Check sheet for the modelled part. Datum: model origin and axes. Units: mm. A direction names the side the tool comes from. Round coordinates to 2 decimals unless told otherwise and drop trailing zeros. Order: outer loops, then holes, each group sorted by start corner. A loop starts at its lowest first (then second) coordinate and runs counter-clockwise, first axis right, second up.
Q1. Cross-section at A-A on y = 2.1. Record the cut outline in (x, z), then the cut area to 3 significant figures.
Q2. Set-up check for faces 4 (the cylindrical face through (-9.534, 2.012, -2.117)), 5 (the flat face through (-6, 0, 9)): record each of +Z, -Z, +X, -X, +Y, -Y from which the full face is reachable in a straight line by a thin tool's end or side.
Q3. Cross-section at B-B on z = 0. Record the cut outline in (x, y).
Q4. Mould release check, pull along X, two halves, no side actions. Record for faces 1 (the cylindrical face through (9.534, 0.616, -2.117)), 2 (the cylindrical face through (-5.205, 1.327, 12.553)), 3 (the flat face through (-9, 2.692, 6)): +X half, -X half, draft (parallel to the pull), parting line (faces both ways), or undercut.
Q5. Depth check by flat-ended pin: P1, Ø6, axis at x = -1, z = 1.5, coming from the -Y side; P2, Ø11.5, axis at x = 0, z = 0, coming from the +Y side. Enter the tip coordinate at first touch or a pass-through.
Q6. Cross-section at C-C on x = 0. Record the cut outline in (y, z), then the cut area to 3 significant figures.
Q7. Cross-section at D-D on x = 12. Record the cut outline in (y, z).
Q8. Scan lines: probe 1 along X at (y, z) = (0.5, 0); probe 2 along Z at (x, y) = (2, 1.45); probe 3 along Z at (x, y) = (4, 1.9). Record each from-to range of solid material in increasing order.
from build123d import *

# Parameters (mm, degrees)
SKETCH1_R           = 13.589
SKETCH1_R_2         = 9.7663
BOSS_EXTRUDE1_DEPTH = 2.6924
SKETCH3_R           = 9.7663
BOSS_EXTRUDE2_DEPTH = 1.35
SKETCH4_R           = 9.7663
CUT_EXTRUDE1_DEPTH  = 1.25


with BuildPart() as part:
    # Sketch1 → Boss-Extrude1 (new body)
    with BuildSketch(Plane(origin=(0, 0, 0), x_dir=(1, 0, 0), z_dir=(0, 1, 0))):
        with Locations(Location((0, 0, 0), (0, 0, 270))):
            Circle(SKETCH1_R)
        with Locations(Location((0, 0, 0), (0, 0, 270))):
            Circle(SKETCH1_R_2, mode=Mode.SUBTRACT)
    extrude(amount=BOSS_EXTRUDE1_DEPTH)

    # Sketch3 → Boss-Extrude2 (add)
    with BuildSketch(Plane(origin=(0, 0, 0), x_dir=(1, 0, 0), z_dir=(0, 1, 0))):
        with Locations(Location((0, 0, 0), (0, 0, 270))):
            Circle(SKETCH3_R)
    extrude(amount=BOSS_EXTRUDE2_DEPTH)

    # Sketch4 → Cut-Extrude1 (cut)
    with BuildSketch(Plane.XZ):
        with Locations(Location((0, 0, 0), (0, 0, 90))):
            Circle(SKETCH4_R)
    extrude(amount=-CUT_EXTRUDE1_DEPTH, mode=Mode.SUBTRACT)


solid = part.part
Results found:
1. outline: circle Ø27.18 at (0, 0); hole circle Ø19.53 at (0, 0)
1. area: 280 mm2
2. face 4: +Y
2. face 5: +Z, -Z, +X, -X, -Y
3. outline: (-13.59, 0) - (-9.77, 0) - (-9.77, 1.25) - (9.77, 1.25) - (9.77, 0) - (13.59, 0) - (13.59, 2.69) - (9.77, 2.69) - (9.77, 1.35) - (-9.77, 1.35) - (-9.77, 2.69) - (-13.59, 2.69) - close
4. face 1: undercut
4. face 2: parting line
4. face 3: draft
5. P1: stops at y = 1.25
5. P2: stops at y = 1.35
6. outline: (0, -13.59) - (2.69, -13.59) - (2.69, -9.77) - (1.35, -9.77) - (1.35, 9.77) - (2.69, 9.77) - (2.69, 13.59) - (0, 13.59) - (0, 9.77) - (1.25, 9.77) - (1.25, -9.77) - (0, -9.77) - close
6. area: 22.5 mm2
7. outline: (0, -6.38) - (2.69, -6.38) - (2.69, 6.38) - (0, 6.38) - close
8. probe 1: x = -13.59 to -9.77, 9.77 to 13.59
8. probe 2: z = -13.44 to -9.56, 9.56 to 13.44
8. probe 3: z = -12.99 to -8.91, 8.91 to 12.99
